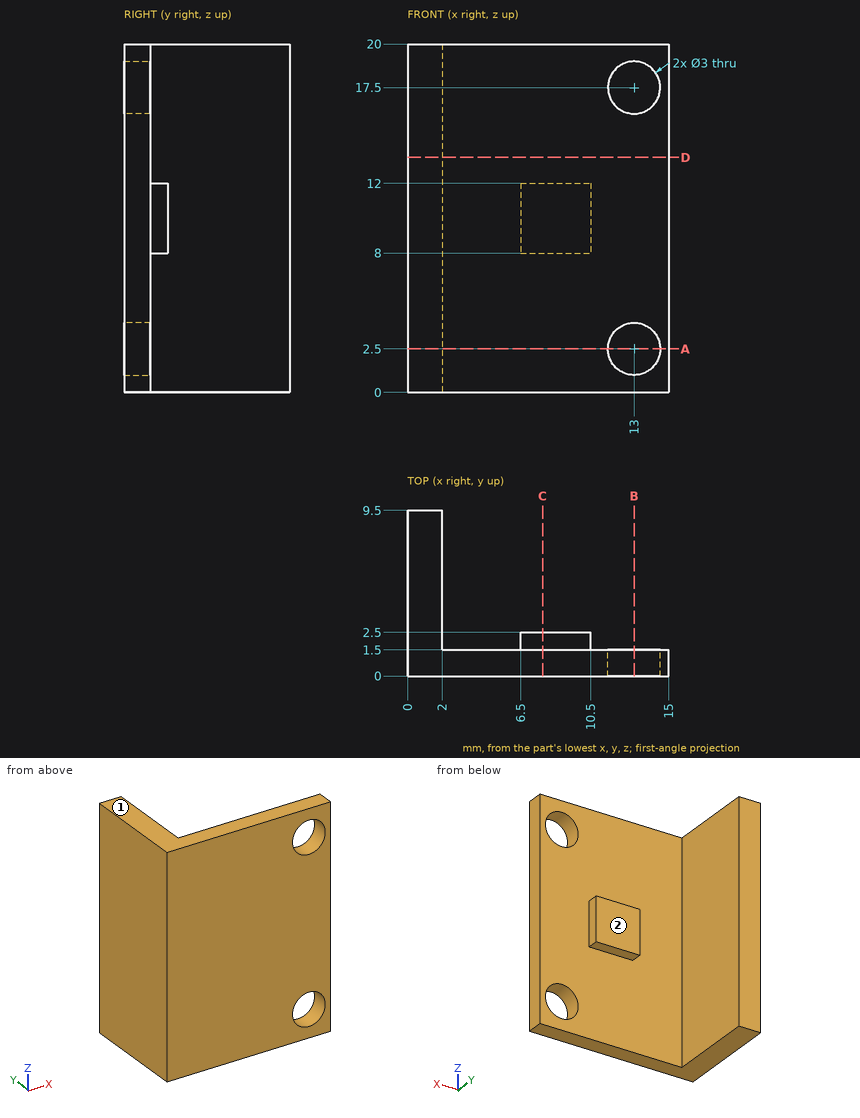
Geometry: see drawing. Coordinates: mm, zero at the bounding-box minimum. A direction names the side the tool comes from. Round coordinates to 2 decimals unless told otherwise and drop trailing zeros. Order: outer loops, then holes, each group sorted by start corner. A loop starts at its lowest first (then second) coordinate and runs counter-clockwise, first axis right, second up. Notation, with made-up numbers: (-5.75, 45.25) - (32.25, 45.25) arc R17 cw to (32.25, 63.25) - close; hole circle Ø5 at (3, 74). An arc over 180 degrees is marked (long way). One line per question, with ' | ' between items. Start each with the question number.
1) Cut plane B-B, the plane x = 13. Return the cut outline in (y, z), then the cut area to 3 significant figures.
2) Set-up query: the marked faces 1 and 2. Return all of +Z, -Z, +X, -X, +Y, -Y with unobstructed straight access to the full face (end or side cutting, diameter ignored); none if empty.
3) Ray query, probe 1 along X at (y, z) = (2, 8.5); probe 2 along X at (y, z) = (0.65, 2.5); probe 3 along Y at (x, z) = (10.75, 3). Return the intervals inside material, ascending.
4) Cut plane D-D, the plane z = 13.5. Return the cut outline in (x, y).
5) Contact query for flat-ended pins moving along their axis: P1, Ø6.5, axis at x = 11, z = 6.5, coming from the +Y side; P2, Ø4, axis at y = 3, z = 9.5, coming from the -X side; P3, Ø2, axis at y = 7.5, z = 4.5, coming from the +X side; P4, Ø0.5, axis at x = 9.5, y = 2, coming from the +Z side. Output: stop coordinate, or through.
6) Cut plane C-C, the plane x = 7.75. Return the cut outline in (y, z).
7) Cut plane A-A, the plane z = 2.5. Return the cut outline in (x, y).
Worked out:
1) outline: (0, 0) - (1.5, 0) - (1.5, 1) - (0, 1) - close; (0, 4) - (1.5, 4) - (1.5, 16) - (0, 16) - close; (0, 19) - (1.5, 19) - (1.5, 20) - (0, 20) - close | area: 21.0 mm^2
2) face 1: +Z, +X, -X, +Y, -Y | face 2: +Z, -Z, +X, +Y
3) probe 1: x = 0 to 2, 6.5 to 10.5 | probe 2: x = 0 to 11.5, 14.5 to 15 | probe 3: y = 0 to 1.5
4) outline: (0, 0) - (15, 0) - (15, 1.5) - (2, 1.5) - (2, 9.5) - (0, 9.5) - close
5) P1: stops at y = 2.5 | P2: stops at x = 0 | P3: stops at x = 2 | P4: stops at z = 12
6) outline: (0, 0) - (1.5, 0) - (1.5, 8) - (2.5, 8) - (2.5, 12) - (1.5, 12) - (1.5, 20) - (0, 20) - close
7) outline: (0, 0) - (11.5, 0) - (11.5, 1.5) - (2, 1.5) - (2, 9.5) - (0, 9.5) - close; (14.5, 0) - (15, 0) - (15, 1.5) - (14.5, 1.5) - close
